Could you check a few things on this model? Use its own coordinates, in mm. Give positions to 0.01 mm unless a question says otherwise; leave off trailing zeros. Loops run counter-clockwise (first coordinate to the right, second up) from the corner with the lowest first, then second, coordinate; pieces in that order, holes last. Notation, with made-up numbers: (30, 47.5) - (52, 47.5) arc R12 ccw to (52, 57.5) - close; hole circle Ø3 at (48.25, 44). An arc over 180 degrees is marked (long way). Write each question's results on one line, items separated by ' | '. Start each with the question number.
1) I'm going to push flat-ended pins straight in: pin 1 (1.5 mm diameter, centred on y = -9, z = 5, fed in from +X) (3 decimals); pin 2 (3 mm diameter, centred on x = 197.5, z = 4.5, fed in from +Y); pin 3 (1 mm diameter, centred on y = -38, z = 1, fed in from -X). Where does each tip first touch, or does it pass through?
2) If I drill on probe 1 along Y at (x, z) = (-72.5, 0.95); probe 2 along Y at (x, z) = (-144, 1.9); probe 3 along Y at (x, z) = (-290.5, 0.3), over which ranges is the centre line in solid material (lowest first)? Write a range as [from, to].
3) I want a section at B-B, the plane z = 1.35. Count the separate pieces of the cut face and the enclosed holes in it, and give its area (3 significant figures).
4) I want a section at C-C, the plane x = -80. Write out the boundary of the cut face in (y, z), and give its area (3 significant figures).
5) I want a section at D-D, the plane x = 100. Write out the boundary of the cut face in (y, z), and give its area (3 significant figures).
6) I want a section at A-A, the plane x = -214.5. Write out the boundary of the cut face in (y, z).
7) If we mould it in two halves opening along X, with no side actions, what happens to faces 1 (the face through (198.65, 67.806, 2.958)), 2 (the face through (175.36, 32.39, 2.96)), 3 (the face through (277.3, 68, 3)), 4 (the face through (-311.797, -68.986, 2.958))? For each: +X half, -X half, draft (parallel to the pull), parting line (faces both ways), or undercut.
from build123d import *

# Parameters (mm, degrees)
F1_DEPTH = 6


with BuildPart() as f1:
    # F0 (on Top) → F1 (new body)
    with BuildSketch(Plane.XY):
        Polygon((-297.5, -55), (-297.5, -75), (-162.5, -75), (-162.5, -25), (-251.5, -25), (-251.5, -22), (-309.5, -22), (-309.5, -39), (-317.5, -39), (-317.5, -55), align=None)
        with BuildLine():
            ThreePointArc((-317.5, -55), (-311.6421356237, -69.1421356237), (-297.5, -75))
            Line((-297.5, -75), (-297.5, -55))
            Line((-297.5, -55), (-317.5, -55))
        make_face()
        with BuildLine():
            Line((-162.5, -25), (-162.5, -75))
            Line((-162.5, -75), (212.5, -75))
            Line((212.5, -75), (212.5, -70))
            Line((212.5, -70), (212.5, -22))
            Line((212.5, -22), (202.5606023011, -22))
            ThreePointArc((202.5606023011, -22), (199.1728742742, -34.9388939069), (188.5, -43))
            Line((188.5, -43), (180.5, -43))
            Line((180.5, -43), (180.5, -25))
            Line((180.5, -25), (148.5, -25))
            Line((148.5, -25), (148.5, -22))
            Line((148.5, -22), (-31.5, -22))
            Line((-31.5, -22), (-31.5, -25))
            Line((-31.5, -25), (-162.5, -25))
        make_face()
        with BuildLine():
            Line((213.5, -70), (213.5, -75))
            Line((213.5, -75), (317.5, -75))
            Line((317.5, -75), (288.1807403902, 50.6539697565))
            ThreePointArc((288.1807403902, 50.6539697565), (277.083392323, 68.1740192438), (257.5, 75))
            Line((257.5, 75), (212.5, 75))
            Line((212.5, 75), (212.5, 53))
            Line((212.5, 53), (212.5, 51.5))
            Line((212.5, 51.5), (212.5, -22))
            Line((212.5, -22), (212.5, -70))
            Line((212.5, -70), (213.5, -70))
        make_face()
        Polygon((-317.5, 11), (-317.5, -5), (-309.5, -5), (-309.5, -22), (-251.5, -22), (-251.5, -19), (-162.5, -19), (-162.5, 31), (-297.5, 31), (-297.5, 11), align=None)
        with BuildLine():
            Line((202.5606023011, -22), (212.5, -22))
            Line((212.5, -22), (212.5, 51.5))
            Line((212.5, 51.5), (191.8430768086, 51.5))
            ThreePointArc((191.8430768086, 51.5), (175.0535129869, 32.1936689306), (150.5, 25))
            Line((150.5, 25), (112.5, 25))
            Line((112.5, 25), (-107.5, 25))
            Line((-107.5, 25), (-107.5, 31))
            Line((-107.5, 31), (-162.5, 31))
            Line((-162.5, 31), (-162.5, -19))
            Line((-162.5, -19), (-31.5, -19))
            Line((-31.5, -19), (-31.5, -22))
            Line((-31.5, -22), (148.5, -22))
            Line((148.5, -22), (148.5, -19))
            Line((148.5, -19), (170.5, -19))
            Line((170.5, -19), (170.5, -4))
            Line((170.5, -4), (176.5, -4))
            ThreePointArc((176.5, -4), (193.8141294499, -6.7978252425), (202.5606023011, -22))
        make_face()
        with BuildLine():
            ThreePointArc((-297.5, 31), (-311.6421356237, 25.1421356237), (-317.5, 11))
            Line((-317.5, 11), (-297.5, 11))
            Line((-297.5, 11), (-297.5, 31))
        make_face()
        Polygon((-107.5, 59), (-162.5, 31), (-107.5, 31), align=None)
        with BuildLine():
            Line((192.5, 53), (212.5, 53))
            Line((212.5, 53), (212.5, 75))
            ThreePointArc((212.5, 75), (198.4968622639, 67.6392161237), (192.5, 53))
        make_face()
        Polygon((180.5, -43), (188.5, -43), (180.5, -25), align=None)
        Polygon((170.5, -19), (176.5, -4), (170.5, -4), align=None)
        with BuildLine():
            Line((-107.5, 59), (-107.5, 31))
            Line((-107.5, 31), (80.5750319553, 31))
            ThreePointArc((80.5750319553, 31), (25.9745832288, 44.5374524252), (-27.5, 62))
            Line((-27.5, 62), (-27.5, 59))
            Line((-27.5, 59), (-107.5, 59))
        make_face()
        with BuildLine():
            Line((80.5750319553, 31), (-107.5, 31))
            Line((-107.5, 31), (-107.5, 25))
            Line((-107.5, 25), (112.5, 25))
            ThreePointArc((112.5, 25), (96.5060750704, 27.8327083402), (80.5750319553, 31))
        make_face()
        with BuildLine():
            ThreePointArc((-101.0171084337, 62), (-104.2866693361, 60.5607557565), (-107.5, 59))
            Line((-107.5, 59), (-27.5, 59))
            Line((-27.5, 59), (-27.5, 62))
            Line((-27.5, 62), (-101.0171084337, 62))
        make_face()
        with BuildLine():
            ThreePointArc((-27.5, 62), (-64.2585542169, 69.3734629996), (-101.0171084337, 62))
            Line((-101.0171084337, 62), (-27.5, 62))
        make_face()
    extrude(amount=F1_DEPTH)


solid = f1.part
Answers:
1) pin 1: stops at x = 302.275 | pin 2: stops at y = 68.18 | pin 3: stops at x = -309.5
2) probe 1: y = [-75, -25], [-19, 69.02] | probe 2: y = [-75, -25], [-19, 40.42] | probe 3: y = [-75, 31]
3) separate pieces: 1 | enclosed holes: 2 | area: 72,100 mm2
4) outline: (-75, 0) - (-25, 0) - (-25, 6) - (-75, 6) - close; (-19, 0) - (68.06, 0) - (68.06, 6) - (-19, 6) - close | area: 822 mm2
5) outline: (-75, 0) - (27.18, 0) - (27.18, 6) - (-75, 6) - close | area: 613 mm2
6) outline: (-75, 0) - (-25, 0) - (-25, 6) - (-75, 6) - close; (-19, 0) - (31, 0) - (31, 6) - (-19, 6) - close
7) face 1: undercut | face 2: undercut | face 3: +X half | face 4: -X half
